Work out the finished part from the listing and answer in its coordinate system (mm). Face numbers are marked on the shaded views. A direction names the side the tool comes from. Round coordinates to 2 decimals unless told otherwise and drop trailing zeros. Order: outer loops, then holes, each group sorted by start corner. A loop starts at its lowest first (then second) coordinate and runs counter-clockwise, first axis right, second up. Notation, with made-up numbers: (89.25, 66.5) - (110.25, 66.5) arc R6 cw to (110.25, 73.5) - close; hole circle Ø9 at (6, 13). An arc over 180 degrees is marked (long way). Answer in a Markdown table with one row per item.
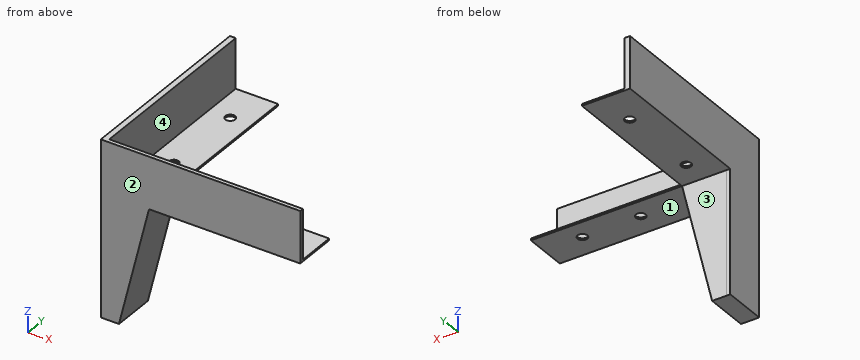
from build123d import *

# Parameters (mm, degrees)
F1_DEPTH  = 2
F2_W      = 2
F2_H      = 76.6198585529
F3_DEPTH  = 20
F4_DEPTH  = 19.9898
F5_W      = 22.560308024
F5_H      = 13.6446189195
F5_W_2    = 2
F6_DEPTH  = 76.2
F7_DEPTH  = 25.4
F9_DEPTH  = 12.7
F10_DEPTH = 12.7
F12_D     = 5


with BuildPart() as f1:
    # F0 (on Front) → F1 (new body)
    with BuildSketch(Plane.XZ):
        Polygon((76.2, 0), (0, 0), (0, -76.6198585529), (9.2363302823, -76.6198585529), (24.560308024, -13.6446189195), (76.2, -13.6446189195), align=None)
    extrude(amount=F1_DEPTH)

    # F2 (on face) → F3 (join)
    with BuildSketch(Plane(origin=(0, 0, 0), x_dir=(-1, 0, 0), z_dir=(0, 1, 0))):
        with Locations((-1, -38.3099292764)):
            Rectangle(F2_W, F2_H)
    extrude(amount=F3_DEPTH)

    # F4 (add): a face of the model
    f4_faces = [f1.faces().sort_by_distance(p)[0] for p in [
        (15.8619650851, 0, -44.8800592008),
    ]]
    extrude(f4_faces, amount=F4_DEPTH)

    # F5 (on face) → F6 (join)
    with BuildSketch(Plane(origin=(0, 19.9898, 0), x_dir=(-1, 0, 0), z_dir=(0, 1, 0))):
        with Locations((-13.280154012, -6.8223094598)):
            Rectangle(F5_W, F5_H)
        with Locations((-1, -6.8223094598)):
            Rectangle(F5_W_2, F5_H)
    extrude(amount=F6_DEPTH)

    # F7 (add): a face of the model
    f7_faces = [f1.faces().sort_by_distance(p)[0] for p in [
        (76.2, 8.9949, -6.8223094598),
    ]]
    extrude(f7_faces, amount=F7_DEPTH)

    # F8 (on face) → F9 (cut)
    with BuildSketch(Plane.XY):
        Polygon((2.9516927898, 0), (101.6, 0), (101.6, 19.9898), (24.560308024, 19.9898), (24.560308024, 96.1898), (2.9516927898, 96.1898), align=None)
    extrude(amount=-F9_DEPTH, mode=Mode.SUBTRACT)

    # F10 (add): a face of the model
    f10_faces = [f1.faces().sort_by_distance(p)[0] for p in [
        (1.412933007, 47.0949, 0),
    ]]
    extrude(f10_faces, amount=F10_DEPTH)

    # F12 (through all)
    with Locations(Plane.XY.offset(-12.7)):
        with Locations((81.9915756583, 9.9949), (52.2758463949, 9.9949), (13.7560004069, 32.9941399395), (13.7560004069, 75.88840276)):
            Hole(F12_D / 2)


solid = f1.part
1) Each of these flat-tipped pins is pushed along its axis until it touches: pin 1 (25 mm diameter, centred on x = 15.5, z = -47.5, fed in from +Y); pin 2 (6 mm diameter, centred on x = 14, y = 56, fed in from +Z); pin 3 (12.5 mm diameter, centred on x = 12.5, y = 48.5, fed in from -Z); pin 4 (4 mm diameter, centred on x = 81.99, y = 9.99, fed in from +Z). Where does it stop, or does it pass through?
Filled in:
| item | result |
|---|---|
| pin 1 | stops at y = 19.99 |
| pin 2 | stops at z = -12.7 |
| pin 3 | stops at z = -13.64 |
| pin 4 | passes through |
2) Find section B-B, the plane z = -1. Give the vertices of the cut face in (x, y), then the cut area to 3 significant figures.
Filled in:
| item | result |
|---|---|
| outline | (0, -2) - (101.6, -2) - (101.6, 0) - (2.95, 0) - (2.95, 96.19) - (0, 96.19) - close |
| area | 487 mm^2 |
3) Find the intervals of material crossed by probe 1 along X at (y, z) = (18, 7); probe 2 along Z at (x, y) = (8, 9.5); probe 3 along Y at (x, z) = (78, 2), in increasing order. Write a range as from..to.
Filled in:
| item | result |
|---|---|
| probe 1 | x = 0..2.95 |
| probe 2 | z = -76.62..-12.7 |
| probe 3 | y = -2..0 |
4) Find section A-A, the plane x = 13. Give the vertices of the cut face in (y, z).
Filled in:
| item | result |
|---|---|
| outline | (-2, -61.15) - (19.99, -61.15) - (19.99, -13.64) - (30.61, -13.64) - (30.61, -12.7) - (0, -12.7) - (0, 12.7) - (-2, 12.7) - close; (35.38, -13.64) - (73.51, -13.64) - (73.51, -12.7) - (35.38, -12.7) - close; (78.27, -13.64) - (96.19, -13.64) - (96.19, -12.7) - (78.27, -12.7) - close |
5) Which of the six approach directions +Z, -Z, +X, -X, +Y, -Y give full straight-line access (tool end or side, diameter ignored) to the marked faces 1, 2, 3 and 4?
Filled in:
| item | result |
|---|---|
| face 1 | -Z, +X, +Y, -Y |
| face 2 | +Z, -Z, +X, -X, -Y |
| face 3 | -Z, +X, -X, +Y |
| face 4 | +Z, +X, +Y |
6) Find section C-C, the plane y = 87.5. Give the vertices of the cut face in (x, z).
Filled in:
| item | result |
|---|---|
| outline | (0, -13.64) - (24.56, -13.64) - (24.56, -12.7) - (2.95, -12.7) - (2.95, 12.7) - (0, 12.7) - close |
7) Find section D-D, the plane x = 53. Give the vertices of the cut face in (y, z), then the cut area to 3 significant figures.
Filled in:
| item | result |
|---|---|
| outline | (-2, -13.64) - (7.6, -13.64) - (7.6, -12.7) - (0, -12.7) - (0, 12.7) - (-2, 12.7) - close; (12.39, -13.64) - (19.99, -13.64) - (19.99, -12.7) - (12.39, -12.7) - close |
| area | 67.1 mm^2 |
